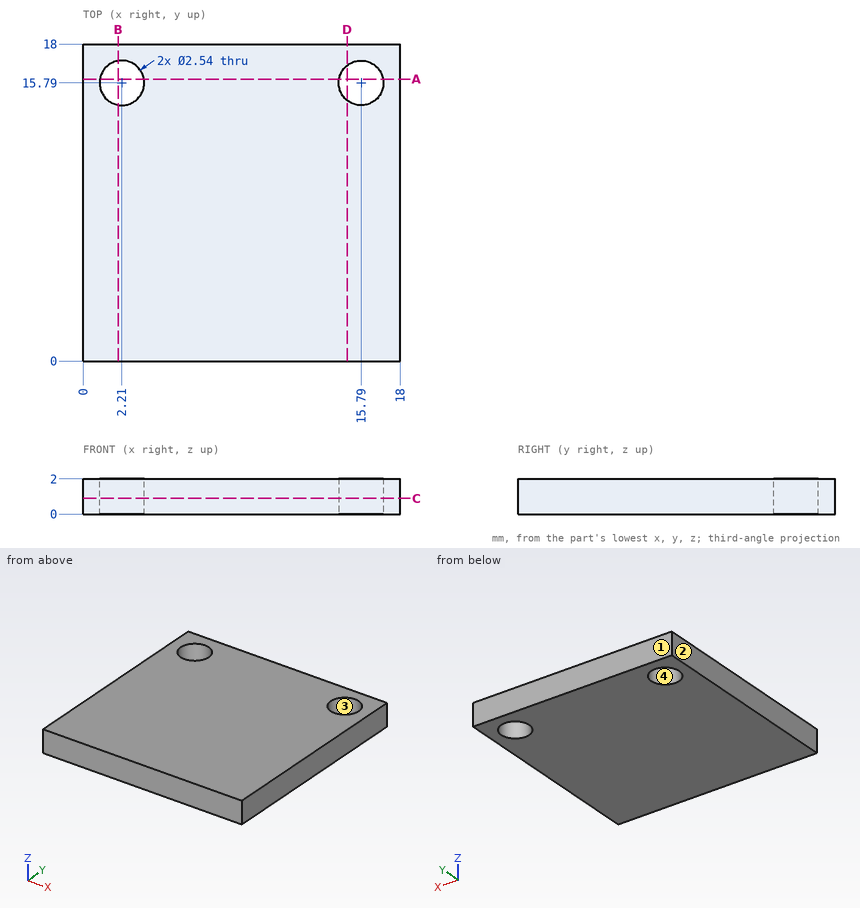
Verification items for this drawing (mm, ordinates from the low corner). Coordinates: 2 decimals unless noted, no trailing zeros. Write each loop counter-clockwise with the first axis right and the second up, starting at its lowest first coordinate (ties: lowest second). Pieces come first, ordered by that corner, then holes. Notation, with made-up numbers: M 34.25,14 L 67.25,14 A18 ccw 67.25,37 Z; hole C 89.5,15.5 d2. An arc over 180 degrees is marked long. Answer as a JSON object with one key per item and string values.
1. Section check B-B, the plane x = 2. Enter the section's corners in (y, z), plus the area to 3 significant figures.
Answers below:
{"outline": "M 0,0 L 14.54,0 L 14.54,2 L 0,2 Z; M 17.04,0 L 18,0 L 18,2 L 17.04,2 Z", "area": "31.0 mm²"}
2. Section check C-C, the plane z = 0.9. Enter the section's corners in (x, y).
Answers below:
{"outline": "M 0,0 L 18,0 L 18,18 L 0,18 Z; hole C 2.21,15.79 d2.54; hole C 15.79,15.79 d2.54"}
3. Draft check along X on the marked faces 1, 2, 3 and 4. Enter one of: released by +X, released by -X, zero draft, split by the parting line, or undercut.
Answers below:
{"face 1": "zero draft", "face 2": "released by -X", "face 3": "undercut", "face 4": "undercut"}
4. Section check A-A, the plane y = 16. Enter the section's corners in (x, z).
Answers below:
{"outline": "M 0,0 L 0.96,0 L 0.96,2 L 0,2 Z; M 3.46,0 L 14.54,0 L 14.54,2 L 3.46,2 Z; M 17.04,0 L 18,0 L 18,2 L 17.04,2 Z"}
5. Scan lines: L1, parallel to X at y = 15.75, z = 0.4; L2, parallel to X at y = 16, z = 1.5; L3, parallel to Y at x = 2.75, z = 1.7. Record each from-to range of solid material in increasing order.
Answers below:
{"L1": "x = 0 to 0.94, 3.48 to 14.52, 17.06 to 18", "L2": "x = 0 to 0.96, 3.46 to 14.54, 17.04 to 18", "L3": "y = 0 to 14.64, 16.94 to 18"}
6. Section check D-D, the plane x = 15. Enter the section's corners in (y, z).
Answers below:
{"outline": "M 0,0 L 14.8,0 L 14.8,2 L 0,2 Z; M 16.78,0 L 18,0 L 18,2 L 16.78,2 Z"}
